from build123d import *

# Parameters (mm, degrees)
EXTRUDE_THIN1_DEPTH = 25.4
CUT_EXTRUDE1_REACH  = 172.75
SKETCH5_RX          = 2.38125
SKETCH5_RY          = 2.381249971
SKETCH5_RX_2        = 1.550642295
SKETCH5_RY_2        = 1.550642276
SKETCH5_RX_3        = 1.646158252
SKETCH5_RY_3        = 1.646158232
FILLET1_R           = 2.54


with BuildPart() as part:
    # Sketch2 → Extrude-Thin1 (new body, symmetric)
    with BuildSketch(Plane(origin=(1981.2, 0, 0), x_dir=(0, 0, -1), z_dir=(1, 0, 0))):
        with BuildLine():
            Line((220.466063539, 151.267804305), (176.948936788, 218.39459013))
            ThreePointArc((176.948936788, 218.39459013), (167.722867176, 224.105285456), (157.452600901, 220.60470947))
            ThreePointArc((157.452600901, 220.60470947), (138.741359143, 55.545453365), (297.061605662, 5.252629462))
            ThreePointArc((297.061605662, 5.252629462), (304.44942683, 13.199484184), (303.002052812, 23.952972457))
            Line((303.002052812, 23.952972457), (274.455306754, 67.987389518))
            Line((274.455306754, 67.987389518), (272.32398896, 66.605693293))
            Line((272.32398896, 66.605693293), (300.870735018, 22.571276232))
            ThreePointArc((300.870735018, 22.571276232), (302.028634232, 13.968485614), (296.118377298, 7.611001836))
            ThreePointArc((296.118377298, 7.611001836), (140.872676937, 56.927149591), (159.220550284, 218.780989377))
            ThreePointArc((159.220550284, 218.780989377), (167.436763304, 221.581450166), (174.817618993, 217.012893905))
            Line((174.817618993, 217.012893905), (218.334745745, 149.88610808))
            Line((218.334745745, 149.88610808), (220.466063539, 151.267804305))
        make_face()
    extrude(amount=EXTRUDE_THIN1_DEPTH, both=True)

    # Sketch5 → Cut-Extrude1 (cut, up to next)
    with BuildSketch(Plane(origin=(0, 145.393223301, -224.274452143), x_dir=(-1, 0, 0), z_dir=(0, 0.543974892, -0.839101494)), mode=Mode.PRIVATE) as cut_extrude1_sk1:
        with Locations(Location((-1997.906331803, -111.078184062), (0, 0, 180))):
            Ellipse(SKETCH5_RX, SKETCH5_RY)
    cut_extrude1_tool1 = extrude(cut_extrude1_sk1.sketch, amount=-CUT_EXTRUDE1_REACH, mode=Mode.PRIVATE) & part.part
    add(cut_extrude1_tool1.solids().sort_by_distance((1997.906332, 52.187353, -284.698195))[0], mode=Mode.SUBTRACT)
    # Sketch5 → Cut-Extrude1 (cut, up to next)
    with BuildSketch(Plane(origin=(0, 145.393223301, -224.274452143), x_dir=(-1, 0, 0), z_dir=(0, 0.543974892, -0.839101494)), mode=Mode.PRIVATE) as cut_extrude1_sk2:
        with Locations(Location((-1963.906331803, -111.078300707), (0, 0, 180))):
            Ellipse(SKETCH5_RX, SKETCH5_RY)
    cut_extrude1_tool2 = extrude(cut_extrude1_sk2.sketch, amount=-CUT_EXTRUDE1_REACH, mode=Mode.PRIVATE) & part.part
    add(cut_extrude1_tool2.solids().sort_by_distance((1963.906332, 52.187255, -284.698259))[0], mode=Mode.SUBTRACT)
    # Sketch5 → Cut-Extrude1 (cut, up to next)
    with BuildSketch(Plane(origin=(0, 145.393223301, -224.274452143), x_dir=(-1, 0, 0), z_dir=(0, 0.543974892, -0.839101494)), mode=Mode.PRIVATE) as cut_extrude1_sk3:
        with Locations(Location((-1967.840481597, -96.661495239), (0, 0, 0))):
            Ellipse(SKETCH5_RX_2, SKETCH5_RY_2)
    cut_extrude1_tool3 = extrude(cut_extrude1_sk3.sketch, amount=-CUT_EXTRUDE1_REACH, mode=Mode.PRIVATE) & part.part
    add(cut_extrude1_tool3.solids().sort_by_distance((1967.840482, 64.284418, -276.855879))[0], mode=Mode.SUBTRACT)
    # Sketch5 → Cut-Extrude1 (cut, up to next)
    with BuildSketch(Plane(origin=(0, 145.393223301, -224.274452143), x_dir=(-1, 0, 0), z_dir=(0, 0.543974892, -0.839101494)), mode=Mode.PRIVATE) as cut_extrude1_sk4:
        with Locations(Location((-1993.656290613, -96.661406671), (0, 0, 0))):
            Ellipse(SKETCH5_RX_3, SKETCH5_RY_3)
    cut_extrude1_tool4 = extrude(cut_extrude1_sk4.sketch, amount=-CUT_EXTRUDE1_REACH, mode=Mode.PRIVATE) & part.part
    add(cut_extrude1_tool4.solids().sort_by_distance((1993.656291, 64.284493, -276.85583))[0], mode=Mode.SUBTRACT)
    # Sketch5 → Cut-Extrude1 (cut, up to next)
    with BuildSketch(Plane(origin=(0, 145.393223301, -224.274452143), x_dir=(-1, 0, 0), z_dir=(0, 0.543974892, -0.839101494)), mode=Mode.PRIVATE) as cut_extrude1_sk5:
        with Locations(Location((-1967.840110504, 11.504920485), (0, 0, 180))):
            Ellipse(SKETCH5_RX_2, SKETCH5_RY_2)
    cut_extrude1_tool5 = extrude(cut_extrude1_sk5.sketch, amount=-CUT_EXTRUDE1_REACH, mode=Mode.PRIVATE) & part.part
    add(cut_extrude1_tool5.solids().sort_by_distance((1967.840111, 155.047019, -218.016064))[0], mode=Mode.SUBTRACT)
    # Sketch5 → Cut-Extrude1 (cut, up to next)
    with BuildSketch(Plane(origin=(0, 145.393223301, -224.274452143), x_dir=(-1, 0, 0), z_dir=(0, 0.543974892, -0.839101494)), mode=Mode.PRIVATE) as cut_extrude1_sk6:
        with Locations(Location((-1993.655919521, 11.505009053), (0, 0, 180))):
            Ellipse(SKETCH5_RX_3, SKETCH5_RY_3)
    cut_extrude1_tool6 = extrude(cut_extrude1_sk6.sketch, amount=-CUT_EXTRUDE1_REACH, mode=Mode.PRIVATE) & part.part
    add(cut_extrude1_tool6.solids().sort_by_distance((1993.65592, 155.047094, -218.016016))[0], mode=Mode.SUBTRACT)
    # Sketch5 → Cut-Extrude1 (cut, up to next)
    with BuildSketch(Plane(origin=(0, 145.393223301, -224.274452143), x_dir=(-1, 0, 0), z_dir=(0, 0.543974892, -0.839101494)), mode=Mode.PRIVATE) as cut_extrude1_sk7:
        with Locations(Location((-1963.90586179, 25.921697621), (0, 0, 180))):
            Ellipse(SKETCH5_RX, SKETCH5_RY)
    cut_extrude1_tool7 = extrude(cut_extrude1_sk7.sketch, amount=-CUT_EXTRUDE1_REACH, mode=Mode.PRIVATE) & part.part
    add(cut_extrude1_tool7.solids().sort_by_distance((1963.905862, 167.144158, -210.173699))[0], mode=Mode.SUBTRACT)
    # Sketch5 → Cut-Extrude1 (cut, up to next)
    with BuildSketch(Plane(origin=(0, 145.393223301, -224.274452143), x_dir=(-1, 0, 0), z_dir=(0, 0.543974892, -0.839101494)), mode=Mode.PRIVATE) as cut_extrude1_sk8:
        with Locations(Location((-1997.90586179, 25.921814267), (0, 0, 180))):
            Ellipse(SKETCH5_RX, SKETCH5_RY)
    cut_extrude1_tool8 = extrude(cut_extrude1_sk8.sketch, amount=-CUT_EXTRUDE1_REACH, mode=Mode.PRIVATE) & part.part
    add(cut_extrude1_tool8.solids().sort_by_distance((1997.905862, 167.144256, -210.173636))[0], mode=Mode.SUBTRACT)

    # Fillet1
    fillet1_edges = [part.edges().sort_by_distance(p)[0] for p in [
        (1955.8, 67.296541405, -273.389647857),
        (1955.8, 150.576956192, -219.400404642),
        (2006.6, 67.296541405, -273.389647857),
        (2006.6, 150.576956192, -219.400404642),
    ]]
    fillet(fillet1_edges, radius=FILLET1_R)


solid = part.part
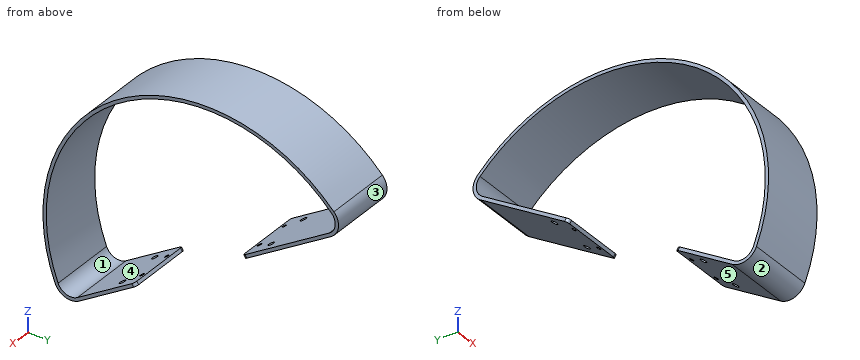
Here's how the part is built. I have some questions about the finished solid (model axes, mm). Face numbers are marked on the shaded views. A direction names the side the tool comes from. Give positions to 0.01 mm unless a question says otherwise; leave off trailing zeros. Loops run counter-clockwise (first coordinate to the right, second up) from the corner with the lowest first, then second, coordinate; pieces in that order, holes last. Notation, with made-up numbers: (-14.75, -25) -> (35.25, -25) arc R32 cw to (35.25, 12) -> close; hole circle Ø5 at (72, 43.25). An arc over 180 degrees is marked (long way). Answer as a JSON object with one key per item and string values. Group by question number.
Item 1: On a 3-axis mill with a long thin cutter (end or side, diameter ignored), from which of +Z, -Z, +X, -X, +Y, -Y can I reach the whole of each face in a straight line? I mean the marked faces 4 and 5. Say none if no direction works.
Item 2: I need wall thicknesses on L1, parallel to Z at x = 2000.5, y = 126.5; L2, parallel to Z at x = 1970, y = 181.5; L3, parallel to Y at x = 1995.5, z = -152. Which ranges of each line are inside material? Lowest first, please.
Item 3: Thinking about a two-plate mould opening in Y: for the marked faces 1, 2 and 3, which applies, pulls with the +Y half, pulls with the -Y half, needs draft (parallel to the pull), parting line crosses it, or undercut?
Item 4: Imagine slicing it at A-A on y = 205. Write out the boundary of the cut face in (x, z).
Item 5: Imagine slicing it at D-D on y = 136.5. Write out the boundary of the cut face in (x, z), then the cut area to 3 significant figures.
Item 6: Imagine slicing it at B-B on z = -184. Write out the boundary of the cut face in (x, y), then the cut area to 3 significant figures.
Item 7: Will these pins go through, and if not, where does the flat tip stop? pin 1 (8 mm diameter, centred on x = 1975, z = -158, fed in from +Y); pin 2 (1.5 mm diameter, centred on x = 1993.5, y = 180.5, fed in from -Z); pin 3 (3 mm diameter, centred on x = 1971, z = -236, fed in from +Y).
Item 8: Imagine slicing it at C-C on z = -228. Write out the boundary of the cut face in (x, y), then the cut area to 3 significant figures.
Answer list:
{
 "1": {"face 4": "+X, -X", "face 5": "-Z, +X, -X, +Y"},
 "2": {"L1": "z = -120.24 to -117.7", "L2": "z = -200.87 to -197.84, -132.54 to -129.73", "L3": "y = 38.4 to 42.2, 211.18 to 214.99"},
 "3": {"face 1": "undercut", "face 2": "parting line crosses it", "face 3": "pulls with the +Y half"},
 "4": {"outline": "(1955.8, -185.63) -> (2006.6, -185.63) -> (2006.6, -182.61) -> (1955.8, -182.61) -> close; (1955.8, -146.92) -> (2006.6, -146.92) -> (2006.6, -143.73) -> (1955.8, -143.73) -> close"},
 "5": {"outline": "(1955.8, -120.61) -> (2006.6, -120.61) -> (2006.6, -118.06) -> (1955.8, -118.06) -> close", "area": "129 mm2"},
 "6": {"outline": "(1955.8, 12.9) -> (2006.6, 12.9) -> (2006.6, 15.83) -> (1955.8, 15.83) -> close; (1955.8, 202.85) -> (2006.6, 202.85) -> (2006.6, 207.52) -> (1955.8, 207.52) -> close", "area": "386 mm2"},
 "7": {"pin 1": "stops at y = 223.44", "pin 2": "stops at z = -202", "pin 3": "stops at y = -0.79"},
 "8": {"outline": "(1955.8, -2.48) -> (2006.6, -2.48) -> (2006.6, 0.09) -> (1955.8, 0.09) -> close", "area": "131 mm2"}
}
